Geometry check sheet. Reference: drawing and pictorial views, mm from the part's lowest x, y, z. Give positions to 0.01 mm unless a question says otherwise; leave off trailing zeros. Write each loop counter-clockwise with the first axis right and the second up, starting at its lowest first coordinate (ties: lowest second). Pieces come first, ordered by that corner, then holes. Notation, with made-up numbers: (5, 6) -> (28, 6) arc R21 cw to (28, 36) -> close; hole circle Ø11 at (40.5, -12.5). An arc over 180 degrees is marked (long way). Use a Markdown table: item, result. Add a question column.
1. Cross-section at B-B (z = 11.25). Enter the section's corners in (x, y).
2. Cross-section at C-C (z = 4). Enter the section's corners in (x, y).
3. Scan lines: probe 1 along Y at (x, z) = (3.5, 21.25); probe 2 along Y at (x, z) = (5.75, 22). Record each from-to range of solid material in increasing order. Write a range as [from, to].
4. Gauge pin test, flat ends, axial feed: P1, Ø3, axis at x = 4.5, z = 20, coming from the -Y side; P2, Ø1.6, axis at x = 4, z = 15.5, coming from the +Y side; P3, Ø1.9, axis at x = 3.5, y = 3.5, coming from the +Z side. Record the tip position at first contact, or that the pin passes through.
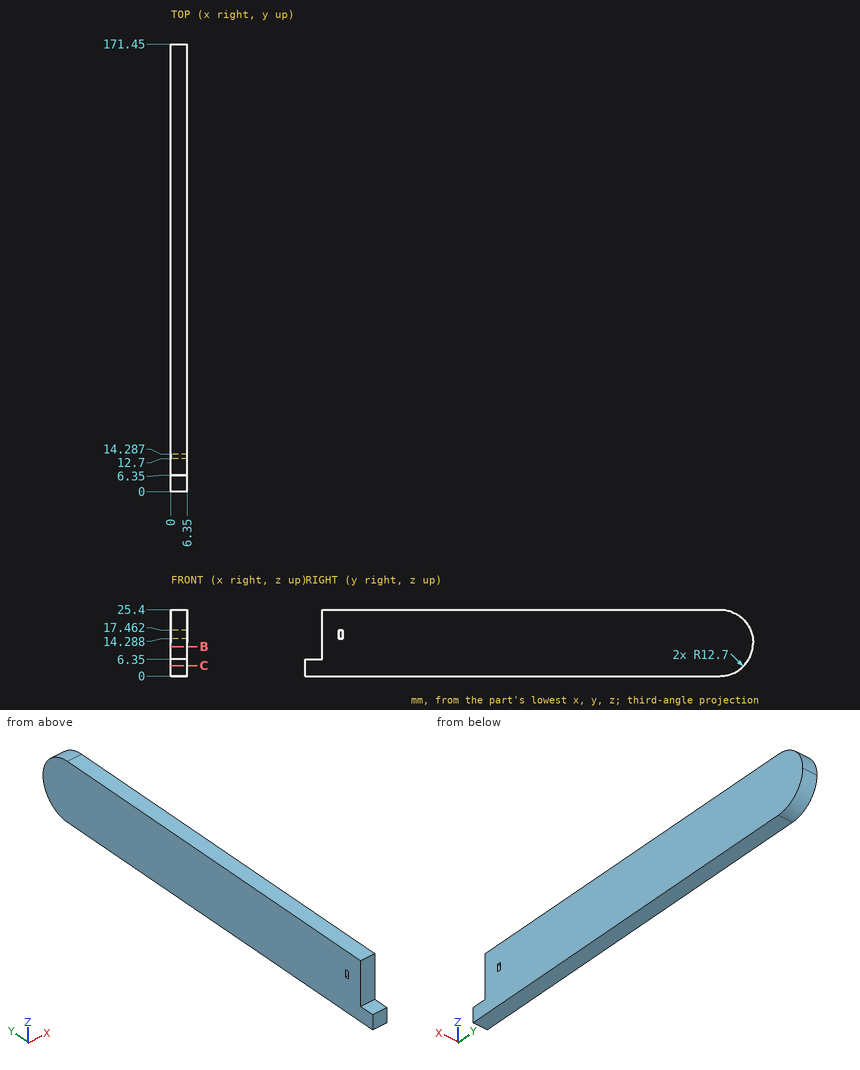
Worked answers:
| question | item | result |
|---|---|---|
| 1 | outline | (0, 6.35) -> (6.35, 6.35) -> (6.35, 171.37) -> (0, 171.37) -> close |
| 2 | outline | (0, 0) -> (6.35, 0) -> (6.35, 168) -> (0, 168) -> close |
| 3 | probe 1 | y = [6.35, 168.14] |
| 3 | probe 2 | y = [6.35, 167.4] |
| 4 | P1 | stops at y = 6.35 |
| 4 | P2 | stops at y = 171.29 |
| 4 | P3 | stops at z = 6.35 |
